from build123d import *

# Parameters (mm, degrees)
CROQUIS1_W              = 84
CROQUIS1_H              = 50
SALIENTE_EXTRUIR1_DEPTH = 5
CORTAR_EXTRUIR5_DEPTH   = 50.132473986
CROQUIS2_R              = 3
CORTAR_EXTRUIR1_DEPTH   = 50.132473986
CROQUIS3_R              = 11
CORTAR_EXTRUIR2_DEPTH   = 2
CROQUIS4_R              = 1.5
CORTAR_EXTRUIR3_DEPTH   = 50.132473986
CROQUIS5_R              = 3.5
CORTAR_EXTRUIR4_DEPTH   = 3
CROQUIS7_W              = 84
CROQUIS7_H              = 4
SALIENTE_EXTRUIR2_DEPTH = 3
REDONDEO1_R             = 3
CHAFL_N1_SIZE           = 1


with BuildPart() as part:
    # Croquis1 → Saliente-Extruir1 (new body)
    with BuildSketch(Plane.XY):
        Rectangle(CROQUIS1_W, CROQUIS1_H)
    extrude(amount=SALIENTE_EXTRUIR1_DEPTH)

    # Croquis6 → Cortar-Extruir5 (cut, through all)
    with BuildSketch(Plane.XY.offset(5)):
        with BuildLine():
            Line((-36, 17), (-26, 17))
            ThreePointArc((-26, 17), (-24, 15), (-26, 13))
            Line((-26, 13), (-36, 13))
            ThreePointArc((-36, 13), (-38, 15), (-36, 17))
        make_face()
        with BuildLine():
            Line((36, 13), (26, 13))
            ThreePointArc((26, 13), (24, 15), (26, 17))
            Line((26, 17), (36, 17))
            ThreePointArc((36, 17), (38, 15), (36, 13))
        make_face()
        with BuildLine():
            Line((36, -17), (26, -17))
            ThreePointArc((26, -17), (24, -15), (26, -13))
            Line((26, -13), (36, -13))
            ThreePointArc((36, -13), (38, -15), (36, -17))
        make_face()
        with BuildLine():
            Line((-36, -13), (-26, -13))
            ThreePointArc((-26, -13), (-24, -15), (-26, -17))
            Line((-26, -17), (-36, -17))
            ThreePointArc((-36, -17), (-38, -15), (-36, -13))
        make_face()
    extrude(amount=-CORTAR_EXTRUIR5_DEPTH, mode=Mode.SUBTRACT)

    # Croquis2 → Cortar-Extruir1 (cut, through all)
    with BuildSketch(Plane.XY.offset(5)):
        Circle(CROQUIS2_R)
    extrude(amount=-CORTAR_EXTRUIR1_DEPTH, mode=Mode.SUBTRACT)

    # Croquis3 → Cortar-Extruir2 (cut)
    with BuildSketch(Plane.XY.offset(5)):
        Circle(CROQUIS3_R)
    extrude(amount=-CORTAR_EXTRUIR2_DEPTH, mode=Mode.SUBTRACT)

    # Croquis4 → Cortar-Extruir3 (cut, through all)
    with BuildSketch(Plane.XY.offset(5)):
        with Locations((15.5, 15.5)):
            Circle(CROQUIS4_R)
        with Locations((-15.5, 15.5)):
            Circle(CROQUIS4_R)
        with Locations((-15.5, -15.5)):
            Circle(CROQUIS4_R)
        with Locations((15.5, -15.5)):
            Circle(CROQUIS4_R)
    extrude(amount=-CORTAR_EXTRUIR3_DEPTH, mode=Mode.SUBTRACT)

    # Croquis5 → Cortar-Extruir4 (cut)
    with BuildSketch(Plane(origin=(0, 0, 0), x_dir=(-1, 0, 0), z_dir=(0, 0, -1))):
        with Locations((-15.5, 15.5)):
            Circle(CROQUIS5_R)
        with Locations((15.5, 15.5)):
            Circle(CROQUIS5_R)
        with Locations((15.5, -15.5)):
            Circle(CROQUIS5_R)
        with Locations((-15.5, -15.5)):
            Circle(CROQUIS5_R)
    extrude(amount=-CORTAR_EXTRUIR4_DEPTH, mode=Mode.SUBTRACT)

    # Croquis7 → Saliente-Extruir2 (add)
    with BuildSketch(Plane.XY.offset(5)):
        with Locations((0, 23)):
            Rectangle(CROQUIS7_W, CROQUIS7_H)
        with Locations((0, -23)):
            Rectangle(CROQUIS7_W, CROQUIS7_H)
    extrude(amount=SALIENTE_EXTRUIR2_DEPTH)

    # Redondeo1
    redondeo1_edges = [part.edges().sort_by_distance(p)[0] for p in [
        (42, -25, 4),
        (-42, -25, 4),
        (-42, 25, 4),
        (42, 25, 4),
    ]]
    fillet(redondeo1_edges, radius=REDONDEO1_R)

    # Chaflán1
    chafl_n1_edges = [part.edges().sort_by_distance(p)[0] for p in [
        (-38, 15, 0),
        (-31, 17, 0),
        (-24, 15, 0),
        (-31, 13, 0),
        (38, 15, 0),
        (31, 13, 0),
        (24, 15, 0),
        (31, 17, 0),
        (38, -15, 0),
        (31, -17, 0),
        (24, -15, 0),
        (31, -13, 0),
        (-38, -15, 0),
        (-31, -13, 0),
        (-24, -15, 0),
        (-31, -17, 0),
    ]]
    chamfer(chafl_n1_edges, length=CHAFL_N1_SIZE)


solid = part.part
Build history of the part. All positions in model axes, mm. A direction names the side the tool comes from. Give positions to 0.01 mm unless a question says otherwise; leave off trailing zeros. Order: outer loops, then holes, each group sorted by start corner. A loop starts at its lowest first (then second) coordinate and runs counter-clockwise, first axis right, second up. Notation, with made-up numbers: M 70,33.25 L 101,33.25 A27 cw 101,63.25 Z; hole C 72.5,5 d11. An arc over 180 degrees is marked long. Put each result on its own line as item: value.
Item 1: Which spindle directions (+Z, -Z, +X, -X, +Y, -Y) get a long thin tool onto all of the face, cutting with end or side? Do faces 1 (the face through (12.16, 16.55, 1.48)), 2 (the face through (-24, 15, 3)), 3 (the face through (-1, -21, 6)). Say none if no direction does.
Results are:
face 1: -Z
face 2: +Z, -Z
face 3: +Z, +X, -X
Item 2: Drop flat-ended pins along their axis: pin 1 Ø2.5 at (x, y) = (-15.5, -15.5) entering from +Z; pin 2 Ø17.5 at (x, y) = (1, 3) entering from +Z; pin 3 Ø5.5 at (x, y) = (-15.5, 15.5) entering from -Z. Give the stop position or say it passes through.
Results are:
pin 1: through
pin 2: z = 5
pin 3: z = 3
Item 3: Wall check: probe 1 along Y at (x, z) = (-15.5, 4.4); probe 2 along Y at (x, z) = (29, 4.75); probe 3 along Y at (x, z) = (-22.5, 6.5). Give the ranges that are in metal, low to high.
Results are:
probe 1: -25 to -17, -14 to 14, 17 to 25
probe 2: -25 to -17, -13 to 13, 17 to 25
probe 3: -25 to -21, 21 to 25
Item 4: Cut at C-C on z = 6.25. Write the cut outline in (x, y).
Results are:
outline: M -42,-22 A3 ccw -39,-25 L 39,-25 A3 ccw 42,-22 L 42,-21 L -42,-21 Z; M -42,21 L 42,21 L 42,22 A3 ccw 39,25 L -39,25 A3 ccw -42,22 Z
Item 5: Cut at D-D on x = 0. Write the cut outline in (y, z), then the cut area to 3 significant figures.
Results are:
outline: M -25,0 L -3,0 L -3,3 L -11,3 L -11,5 L -21,5 L -21,8 L -25,8 Z; M 3,0 L 25,0 L 25,8 L 21,8 L 21,5 L 11,5 L 11,3 L 3,3 Z
area: 212 mm2
Item 6: Cut at B-B on x = -35. Write the cut outline in (y, z).
Results are:
outline: M -25,0 L -18,0 L -17,1 L -17,5 L -21,5 L -21,8 L -25,8 Z; M -13,1 L -12,0 L 12,0 L 13,1 L 13,5 L -13,5 Z; M 17,1 L 18,0 L 25,0 L 25,8 L 21,8 L 21,5 L 17,5 Z
Item 7: Cut at A-A on y = 0. Write the cut outline in (x, z).
Results are:
outline: M -42,0 L -3,0 L -3,3 L -11,3 L -11,5 L -42,5 Z; M 3,0 L 42,0 L 42,5 L 11,5 L 11,3 L 3,3 Z
Item 8: Pull direction Y, two halves, no side cores. Call faces 4 (the face through (-3, 0, 2)), 5 (the face through (41.14, -24.1, 3.94)), 6 (the face through (-41.14, 24.1, 3.94)): +Y half, -Y half, draft (parallel to the pull), parting line (faces both ways), or undercut.
Results are:
face 4: undercut
face 5: -Y half
face 6: +Y half
